Geometry: final body of the model. Coordinates: model frame, mm. A direction names the side the tool comes from. Round coordinates to 2 decimals unless told otherwise and drop trailing zeros. Loops run counter-clockwise (first coordinate to the right, second up) from the corner with the lowest first, then second, coordinate; pieces in that order, holes last. Notation, with made-up numbers: M 0.5,40.25 L 54.5,40.25 A29 cw 54.5,75.25 Z; hole C -27.75,-39 d2. An arc over 180 degrees is marked long. Return JSON: item names as keys, results as strings.
from build123d import *

# Parameters (mm, degrees)
SKETCH1_R                     = 1
BOSS_EXTRUDE1_DEPTH           = 3.4
BOSS_EXTRUDE3_DEPTH           = 5
SKETCH4_R                     = 1.85
CUT_EXTRUDE1_DEPTH            = 5
SKETCH9_R                     = 19
CENTER_HOLE_DEPTH             = 36.651928419
SKETCH2_R                     = 21.5
SKETCH2_R_2                   = 15
BOSS_EXTRUDE2_DEPTH           = 29.1
SKETCH27_R                    = 0.8
TOP_FACE_MOUNTING_HOLES_DEPTH = 46.247209859
CUT_EXTRUDE17_DEPTH           = 43.205568353
CUT_EXTRUDE10_DEPTH           = 41.360748259
CIRPATTERN3_COUNT             = 4
FILLET8_START                 = -1
FILLET8_DEPTH                 = 9.4


with BuildPart() as part:
    # Sketch1 → Boss-Extrude1 (new body)
    with BuildSketch(Plane(origin=(0, 0, 0), x_dir=(1, 0, 0), z_dir=(0, 1, 0))):
        with BuildLine():
            Line((9.283856957, 24.5), (-9.283856957, 24.5))
            ThreePointArc((-9.283856957, 24.5), (-18.526197667, 18.526197667), (-24.5, 9.283856957))
            Line((-24.5, 9.283856957), (-24.5, -9.283856957))
            ThreePointArc((-24.5, -9.283856957), (-18.526197667, -18.526197667), (-9.283856957, -24.5))
            Line((-9.283856957, -24.5), (9.283856957, -24.5))
            ThreePointArc((9.283856957, -24.5), (18.526197667, -18.526197667), (24.5, -9.283856957))
            Line((24.5, -9.283856957), (24.5, 9.283856957))
            ThreePointArc((24.5, 9.283856957), (18.526197667, 18.526197667), (9.283856957, 24.5))
        make_face()
        with Locations(Location((-13.432490209, 21.084786145, 0), (0, 0, 270))):
            Circle(SKETCH1_R, mode=Mode.SUBTRACT)
        with Locations(Location((-17.67766953, 17.67766953, 0), (0, 0, 270))):
            Circle(SKETCH1_R, mode=Mode.SUBTRACT)
        with Locations(Location((-21.084786145, 13.432490209, 0), (0, 0, 90))):
            Circle(SKETCH1_R, mode=Mode.SUBTRACT)
        with Locations(Location((21.084786145, 13.432490209, 0), (0, 0, 270))):
            Circle(SKETCH1_R, mode=Mode.SUBTRACT)
        with Locations(Location((17.67766953, 17.67766953, 0), (0, 0, 270))):
            Circle(SKETCH1_R, mode=Mode.SUBTRACT)
        with Locations(Location((13.432490209, 21.084786145, 0), (0, 0, 90))):
            Circle(SKETCH1_R, mode=Mode.SUBTRACT)
        with Locations(Location((13.432490209, -21.084786145, 0), (0, 0, 270))):
            Circle(SKETCH1_R, mode=Mode.SUBTRACT)
        with Locations(Location((17.67766953, -17.67766953, 0), (0, 0, 270))):
            Circle(SKETCH1_R, mode=Mode.SUBTRACT)
        with Locations(Location((21.084786145, -13.432490209, 0), (0, 0, 90))):
            Circle(SKETCH1_R, mode=Mode.SUBTRACT)
        with Locations(Location((-21.084786145, -13.432490209, 0), (0, 0, 270))):
            Circle(SKETCH1_R, mode=Mode.SUBTRACT)
        with Locations(Location((-17.67766953, -17.67766953, 0), (0, 0, 270))):
            Circle(SKETCH1_R, mode=Mode.SUBTRACT)
        with Locations(Location((-13.432490209, -21.084786145, 0), (0, 0, 90))):
            Circle(SKETCH1_R, mode=Mode.SUBTRACT)
    extrude(amount=BOSS_EXTRUDE1_DEPTH)

    # Sketch3 → Boss-Extrude3 (add)
    with BuildSketch(Plane(origin=(0, 3.4, 0), x_dir=(1, 0, 0), z_dir=(0, 1, 0))):
        with BuildLine():
            Line((-24.5, 4.974937186), (-24.5, -4.974937186))
            ThreePointArc((-24.5, -4.974937186), (-17.67766953, -17.67766953), (-4.974937186, -24.5))
            Line((-4.974937186, -24.5), (4.974937186, -24.5))
            ThreePointArc((4.974937186, -24.5), (17.67766953, -17.67766953), (24.5, -4.974937186))
            Line((24.5, -4.974937186), (24.5, 4.974937186))
            ThreePointArc((24.5, 4.974937186), (17.67766953, 17.67766953), (4.974937186, 24.5))
            Line((4.974937186, 24.5), (-4.974937186, 24.5))
            ThreePointArc((-4.974937186, 24.5), (-17.67766953, 17.67766953), (-24.5, 4.974937186))
        make_face()
    extrude(amount=BOSS_EXTRUDE3_DEPTH)

    # Sketch4 → Cut-Extrude1 (cut)
    with BuildSketch(Plane(origin=(0, 8.4, 0), x_dir=(1, 0, 0), z_dir=(0, 1, 0))):
        with Locations((-17.67766953, 17.67766953)):
            Circle(SKETCH4_R)
        with Locations((-13.432490209, 21.084786145)):
            Circle(SKETCH4_R)
        with Locations((-21.084786145, 13.432490209)):
            Circle(SKETCH4_R)
        with Locations((21.084786145, 13.432490209)):
            Circle(SKETCH4_R)
        with Locations((17.67766953, 17.67766953)):
            Circle(SKETCH4_R)
        with Locations((13.432490209, 21.084786145)):
            Circle(SKETCH4_R)
        with Locations((13.432490209, -21.084786145)):
            Circle(SKETCH4_R)
        with Locations((17.67766953, -17.67766953)):
            Circle(SKETCH4_R)
        with Locations((21.084786145, -13.432490209)):
            Circle(SKETCH4_R)
        with Locations((-21.084786145, -13.432490209)):
            Circle(SKETCH4_R)
        with Locations((-13.432490209, -21.084786145)):
            Circle(SKETCH4_R)
        with Locations((-17.67766953, -17.67766953)):
            Circle(SKETCH4_R)
    extrude(amount=-CUT_EXTRUDE1_DEPTH, mode=Mode.SUBTRACT)

    # Sketch9 → Center Hole (cut, through all)
    with BuildSketch(Plane(origin=(0, 8.4, 0), x_dir=(1, 0, 0), z_dir=(0, 1, 0))):
        with Locations(Location((0, 0, 0), (0, 0, 270))):
            Circle(SKETCH9_R)
    extrude(amount=-CENTER_HOLE_DEPTH, mode=Mode.SUBTRACT)

    # Sketch2 → Boss-Extrude2 (add)
    with BuildSketch(Plane(origin=(0, 29.1, 0), x_dir=(-1, 0, 0), z_dir=(0, 1, 0))):
        with Locations(Location((0, 0, 0), (0, 0, 90))):
            Circle(SKETCH2_R)
        with Locations(Location((0, 0, 0), (0, 0, 90))):
            Circle(SKETCH2_R_2, mode=Mode.SUBTRACT)
    extrude(amount=-BOSS_EXTRUDE2_DEPTH)

    # Sketch27 → Top Face Mounting Holes (cut, through all)
    with BuildSketch(Plane(origin=(0, 29.1, 0), x_dir=(1, 0, 0), z_dir=(0, 1, 0))):
        with Locations(Location((-16.643489035, 5.407797402, 0), (0, 0, 270))):
            Circle(SKETCH27_R)
        with Locations(Location((-16.643489035, -5.407797402, 0), (0, 0, 90))):
            Circle(SKETCH27_R)
        with Locations(Location((16.643489035, -5.407797402, 0), (0, 0, 270))):
            Circle(SKETCH27_R)
        with Locations(Location((16.643489035, 5.407797402, 0), (0, 0, 90))):
            Circle(SKETCH27_R)
    extrude(amount=-TOP_FACE_MOUNTING_HOLES_DEPTH, mode=Mode.SUBTRACT)

    # Sketch28 → Cut-Extrude17 (cut, through all)
    with BuildSketch(Plane(origin=(0, 24.1, 0), x_dir=(1, 0, 0), z_dir=(0, 1, 0))):
        Polygon((-31.516845347, 27.27420466), (27.27420466, -31.516845347), (31.516845347, -27.27420466), (-27.27420466, 31.516845347), align=None)
    extrude(amount=-CUT_EXTRUDE17_DEPTH, mode=Mode.SUBTRACT)

    # Sketch22 → Cut-Extrude10 (cut, symmetric)
    with BuildSketch(Plane(origin=(0, 8.4, 0), x_dir=(1, 0, 0), z_dir=(0, 1, 0))):
        with BuildLine():
            Line((8, 24.5), (-8, 24.5))
            Line((-8, 24.5), (-8, 22))
            ThreePointArc((-8, 22), (-7.414213562, 20.585786438), (-6, 20))
            Line((-6, 20), (6, 20))
            ThreePointArc((6, 20), (7.414213562, 20.585786438), (8, 22))
            Line((8, 22), (8, 24.5))
        make_face()
    cut_extrude10 = extrude(amount=CUT_EXTRUDE10_DEPTH, both=True, mode=Mode.SUBTRACT)

    # CirPattern3: Cut-Extrude10 ×4 about axis
    cirpattern3_axis = Axis((0, 0, 0), (0, 1, 0))
    for i in range(1, CIRPATTERN3_COUNT):
        add(cut_extrude10.rotate(cirpattern3_axis, i * 360 / CIRPATTERN3_COUNT), mode=Mode.SUBTRACT)

    # Fillet8: read off the stored shape, not the designer's step
    # Fillet8 outline → Fillet8 (cut)
    with BuildSketch(Plane(origin=(0, 0, 0), x_dir=(1, 0, 0), z_dir=(0, 1, 0)).offset(FILLET8_START)):
        with BuildLine():
            Line((24.5, 8), (24.5, 9.283856957))
            ThreePointArc((24.5, 9.283856957), (23.765685797, 8.351927476), (22.632611679, 8))
            Line((22.632611679, 8), (24.5, 8))
        make_face()
        with BuildLine():
            Line((24.5, -8), (22.632611679, -8))
            ThreePointArc((22.632611679, -8), (23.765685797, -8.351927476), (24.5, -9.283856957))
            Line((24.5, -9.283856957), (24.5, -8))
        make_face()
        with BuildLine():
            Line((8, -24.5), (9.283856957, -24.5))
            ThreePointArc((9.283856957, -24.5), (8.351927476, -23.765685797), (8, -22.632611679))
            Line((8, -22.632611679), (8, -24.5))
        make_face()
        with BuildLine():
            Line((-8, -24.5), (-8, -22.632611679))
            ThreePointArc((-8, -22.632611679), (-8.351927476, -23.765685797), (-9.283856957, -24.5))
            Line((-9.283856957, -24.5), (-8, -24.5))
        make_face()
        with BuildLine():
            Line((-24.5, -8), (-24.5, -9.283856957))
            ThreePointArc((-24.5, -9.283856957), (-23.765685797, -8.351927476), (-22.632611679, -8))
            Line((-22.632611679, -8), (-24.5, -8))
        make_face()
        with BuildLine():
            Line((-24.5, 8), (-22.632611679, 8))
            ThreePointArc((-22.632611679, 8), (-23.765685797, 8.351927476), (-24.5, 9.283856957))
            Line((-24.5, 9.283856957), (-24.5, 8))
        make_face()
        with BuildLine():
            Line((8, 24.5), (8, 22.632611679))
            ThreePointArc((8, 22.632611679), (8.351927476, 23.765685797), (9.283856957, 24.5))
            Line((9.283856957, 24.5), (8, 24.5))
        make_face()
        with BuildLine():
            Line((-8, 24.5), (-9.283856957, 24.5))
            ThreePointArc((-9.283856957, 24.5), (-8.351927476, 23.765685797), (-8, 22.632611679))
            Line((-8, 22.632611679), (-8, 24.5))
        make_face()
    extrude(amount=FILLET8_DEPTH, mode=Mode.SUBTRACT)


solid = part.part
Q1. Section query D-D (y = 25). Output: boundary loops of the cut face in (x, z), plus the area to 3 significant figures.
Determined:
{"outline": "M -20.31,-7.06 A21.5 ccw -7.06,-20.31 A2 cw -6,-20 L 6,-20 A2 cw 7.06,-20.31 A21.5 ccw 20.31,-7.06 A2 cw 20,-6 L 20,6 A2 cw 20.31,7.06 A21.5 ccw 7.06,20.31 A2 cw 6,20 L -6,20 A2 cw -7.06,20.31 A21.5 ccw -20.31,7.06 A2 cw -20,6 L -20,-6 A2 cw Z; hole C -16.64,-5.41 d1.6; hole C -16.64,5.41 d1.6; hole C 0,0 d30; hole C 16.64,-5.41 d1.6; hole C 16.64,5.41 d1.6", "area": "676 mm^2"}
Q2. Reachability of faces 1 (the cylindrical face through (-15.298, 18.895, 15.107)), 2 (the flat face through (0, 15, 20)), 3 (the flat face through (10, 8.4, 20)) from +Z, -Z, +X, -X, +Y, -Y: full face, straight path, thin tool, end or side. Return the list, or none.
Determined:
{"face 1": "+Z, -X, +Y", "face 2": "+Z, +Y, -Y", "face 3": "+Z, +X, +Y"}
Q3. Pull-direction query (X, two-part tool) for faces 4 (the flat face through (-20, 8.4, -10)), 5 (the cylindrical face through (-19.546, 5.935, -12.405)), 6 (the cylindrical face through (20.2, 11.52, -6.87)), 7 (the cylindrical face through (-20.18, 11.52, -6.83)); classes: pulls with the +X half, pulls with the -X half, needs draft (parallel to the pull), parting line crosses it, or undercut.
Determined:
{"face 4": "needs draft", "face 5": "undercut", "face 6": "pulls with the +X half", "face 7": "pulls with the -X half"}
Q4. Section query C-C (x = 0). Output: boundary loops of the cut face in (y, z).
Determined:
{"outline": "M 0,-20 L 29.1,-20 L 29.1,-15 L 0,-15 Z; M 0,15 L 29.1,15 L 29.1,20 L 0,20 Z"}
Q5. Section query B-B (y = 12.5). Output: boundary loops of the cut face in (x, z), plus the area to 3 significant figures.
Determined:
{"outline": "M -20.31,-7.06 A21.5 ccw -17.18,-12.93 L -12.51,-8.27 A15 cw 8.27,12.51 L 12.93,17.18 A21.5 ccw 7.06,20.31 A2 cw 6,20 L -6,20 A2 cw -7.06,20.31 A21.5 ccw -20.31,7.06 A2 cw -20,6 L -20,-6 A2 cw Z; M -12.93,-17.18 A21.5 ccw -7.06,-20.31 A2 cw -6,-20 L 6,-20 A2 cw 7.06,-20.31 A21.5 ccw 20.31,-7.06 A2 cw 20,-6 L 20,6 A2 cw 20.31,7.06 A21.5 ccw 17.18,12.93 L 12.51,8.27 A15 cw -8.27,-12.51 Z; hole C -16.64,-5.41 d1.6; hole C -16.64,5.41 d1.6; hole C 16.64,-5.41 d1.6; hole C 16.64,5.41 d1.6", "area": "597 mm^2"}
Q6. Section query A-A (z = 0). Output: boundary loops of the cut face in (x, y), plus the area to 3 significant figures.
Determined:
{"outline": "M -20,0 L -15,0 L -15,29.1 L -20,29.1 Z; M 15,0 L 20,0 L 20,29.1 L 15,29.1 Z", "area": "291 mm^2"}
Q7. Material intervals for L1, parallel to X at y = 8, z = 0; L2, parallel to Z at x = 1, y = 16.25; L3, parallel to Z at x = -16.5, y = 22, sorted ascending.
Determined:
{"L1": "x = -20 to -15, 15 to 20", "L2": "z = -20 to -14.97, 14.97 to 20", "L3": "z = -12.26 to -6.19, -4.62 to 4.62, 6.19 to 13.78"}
Q8. Pin query (flat end, axial travel): pin 1 (3 mm diameter, centred on x = -12.5, z = -20.5, fed in from +Y); pin 2 (6 mm diameter, centred on y = 4, z = -6, fed in from +X); pin 3 (4 mm diameter, centred on y = 22, z = 15, fed in from -X); pin 4 (1.2 mm diameter, centred on x = 17.68, z = -17.68, fed in from +Y). Return the tip coordinate at first contact, or that it passes through.
Determined:
{"pin 1": "stops at y = 8.4", "pin 2": "stops at x = 24.33", "pin 3": "stops at x = -17.12", "pin 4": "passes through"}
